```python
from build123d import *

# Parameters (mm, degrees)
ESBO_O1_R                = 1.65
ESBO_O1_R_2              = 1.5
RESSALTO_EXTRUS_O1_DEPTH = 3


with BuildPart() as part:
    # Esboço1 → Ressalto-extrusão1 (new body)
    with BuildSketch(Plane.XY):
        with BuildLine():
            Line((-92.5, -20.5), (-85, -20.5))
            ThreePointArc((-85, -20.5), (-82.878679656, -19.621320344), (-82, -17.5))
            Line((-82, -17.5), (-82, -13))
            ThreePointArc((-82, -13), (-81.121320344, -10.878679656), (-79, -10))
            Line((-79, -10), (0, -10))
            Line((0, -10), (0, -7.5))
            Line((0, -7.5), (-79, -7.5))
            ThreePointArc((-79, -7.5), (-81.121320344, -6.621320344), (-82, -4.5))
            Line((-82, -4.5), (-82, 4.5))
            ThreePointArc((-82, 4.5), (-81.121320344, 6.621320344), (-79, 7.5))
            Line((-79, 7.5), (0, 7.5))
            Line((0, 7.5), (0, 10))
            Line((0, 10), (-79, 10))
            ThreePointArc((-79, 10), (-81.121320344, 10.878679656), (-82, 13))
            Line((-82, 13), (-82, 17.5))
            ThreePointArc((-82, 17.5), (-82.878679656, 19.621320344), (-85, 20.5))
            Line((-85, 20.5), (-92.5, 20.5))
            ThreePointArc((-92.5, 20.5), (-95.397777479, 18.276457135), (-94, 14.901923789))
            Line((-94, 14.901923789), (-88, 11.437822174))
            ThreePointArc((-88, 11.437822174), (-86.901923789, 10.339745962), (-86.5, 8.839745962))
            Line((-86.5, 8.839745962), (-86.5, -8.839745962))
            ThreePointArc((-86.5, -8.839745962), (-86.901923789, -10.339745962), (-88, -11.437822174))
            Line((-88, -11.437822174), (-94, -14.901923789))
            ThreePointArc((-94, -14.901923789), (-95.397777479, -18.276457135), (-92.5, -20.5))
        make_face()
        with Locations((-92.5, 17.5)):
            Circle(ESBO_O1_R, mode=Mode.SUBTRACT)
        with Locations((-92.5, -17.5)):
            Circle(ESBO_O1_R, mode=Mode.SUBTRACT)
        with Locations((-85, 17.5)):
            Circle(ESBO_O1_R_2, mode=Mode.SUBTRACT)
        with Locations((-85, -17.5)):
            Circle(ESBO_O1_R_2, mode=Mode.SUBTRACT)
    ressalto_extrus_o1 = extrude(amount=RESSALTO_EXTRUS_O1_DEPTH)

    # Espelhar1: Ressalto-extrusão1 across plane
    add(ressalto_extrus_o1.mirror(Plane(origin=(0, 0, 0), x_dir=(0, 0, 1), z_dir=(1, 0, 0))))


solid = part.part
```
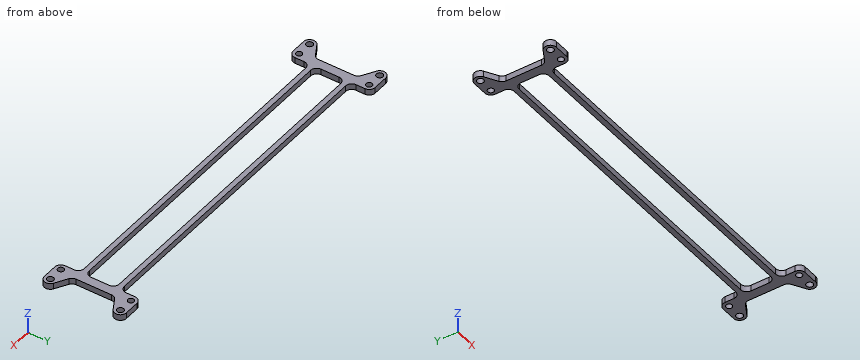
Input: part model. Units: mm. Frame: model coordinates. Give positions to 0.01 mm unless a question says otherwise; leave off trailing zeros. Loops run counter-clockwise (first coordinate to the right, second up) from the corner with the lowest first, then second, coordinate; pieces in that order, holes last.
1) Section query A-A on x = -39.5. Return the cut outline in (y, z).
A:
outline: (-10, 0) - (-7.5, 0) - (-7.5, 3) - (-10, 3) - close; (7.5, 0) - (10, 0) - (10, 3) - (7.5, 3) - close
2) Line query: L1, parallel to Y at x = -6, z = 1.1; L2, parallel to Y at x = -85, z = 1; L3, parallel to X at y = 4.5, z = 2.95. Output: solid intervals per line, ascending.
A:
L1: y = -10 to -7.5, 7.5 to 10
L2: y = -20.5 to -19, -16 to 16, 19 to 20.5
L3: x = -86.5 to -82, 82 to 86.5
3) Section query B-B on y = -1. Return the cut outline in (x, z).
A:
outline: (-86.5, 0) - (-82, 0) - (-82, 3) - (-86.5, 3) - close; (82, 0) - (86.5, 0) - (86.5, 3) - (82, 3) - close
4) Section query C-C on z = 1.5. Count the separate pieces of the cut face and the enclosed holes in it, and give its area (3 significant figures).
A:
separate pieces: 1
enclosed holes: 9
area: 1,390 mm2
5) Contact query for flat-ended pins moving along their axis: pin 1 (2 mm diameter, centred on x = 92.5, y = -17.5, fed in from -Z); pin 2 (1.5 mm diameter, centred on x = 27, z = 1, fed in from +Y); pin 3 (1.5 mm diameter, centred on y = 15, z = 2, fed in from +X); pin 4 (1.5 mm diameter, centred on y = 0, z = 1.5, fed in from -X). Output: stop coordinate, or through.
A:
pin 1: passes through
pin 2: stops at y = 10
pin 3: stops at x = 94.94
pin 4: stops at x = -86.5
